```python
from build123d import *

# Parameters (mm, degrees)
F0_W     = 30
F0_H     = 5
F1_DEPTH = 40
F3_DEPTH = 25


with BuildPart() as f1:
    # F0 (on Top) → F1 (new body)
    with BuildSketch(Plane.XY):
        Polygon((0, 15.2), (0, 0), (76, 0), (76, 5), (76, 10.2), (76, 15.2), align=None)
        with Locations((91, 12.7)):
            Rectangle(F0_W, F0_H)
        with Locations((91, 2.5)):
            Rectangle(F0_W, F0_H)
    extrude(amount=F1_DEPTH)

    # F2 (on face) → F3 (cut)
    with BuildSketch(Plane.XZ):
        with BuildLine():
            ThreePointArc((5.95, 20), (5.2324116139, 21.7324116139), (3.5, 22.45))
            Line((3.5, 22.45), (3.5, 17.55))
            ThreePointArc((3.5, 17.55), (5.2324116139, 18.2675883861), (5.95, 20))
        make_face()
        with BuildLine():
            Line((3.5, 17.55), (3.5, 22.45))
            ThreePointArc((3.5, 22.45), (1.05, 20), (3.5, 17.55))
        make_face()
    extrude(amount=-F3_DEPTH, mode=Mode.SUBTRACT)


solid = f1.part
```
CAD build for the part. Positions are in the model's coordinates, mm. A direction names the side the tool comes from. Coordinates: 2 decimals unless noted, no trailing zeros. Write each loop counter-clockwise with the first axis right and the second up, starting at its lowest first coordinate (ties: lowest second). Pieces come first, ordered by that corner, then holes.
(1) 3-axis set-ups, long thin cutter, end or side, ignore diameter. For faces 1 (the face through (76, 8, 20)), 2 (the face through (54, 15.2, 20)): which of +Z, -Z, +X, -X, +Y, -Y reach the whole face in a straight line?
(2) Two-plate mould, pull along Y, no slides. Class faces 3 (the face through (91, 10.2, 20)), 4 (the face through (52, 8, 0)), 5 (the face through (52, 0, 20)): +Y half, -Y half, draft (parallel to the pull), parting line (faces both ways), or undercut.
(3) Cut at A-A, the plane z = 10.5. List the corners of the cut face in (x, y), and give its area (3 significant figures).
(4) Drill centre lines: probe 1 along Y at (x, z) = (89, 6); probe 2 along X at (y, z) = (6.5, 26); probe 3 along Z at (x, y) = (5, 14.75). Where is each one in solid material? Low to high.
Geometry says:
1. face 1: +Z, -Z, +X
1. face 2: +Z, -Z, +X, -X, +Y
2. face 3: undercut
2. face 4: draft
2. face 5: -Y half
3. outline: (0, 0) - (106, 0) - (106, 5) - (76, 5) - (76, 10.2) - (106, 10.2) - (106, 15.2) - (0, 15.2) - close
3. area: 1,460 mm2
4. probe 1: y = 0 to 5, 10.2 to 15.2
4. probe 2: x = 0 to 76
4. probe 3: z = 0 to 18.06, 21.94 to 40
